Geometry check sheet. Reference: the model listing, model coordinates, mm. Face numbers are marked on the shaded views. A direction names the side the tool comes from. Coordinates: 2 decimals unless noted, no trailing zeros. Order: outer loops, then holes, each group sorted by start corner. A loop starts at its lowest first (then second) coordinate and runs counter-clockwise, first axis right, second up. Notation, with made-up numbers: M 65.25,-16.75 L 101.25,-16.75 A32 ccw 101.25,12.25 Z; hole C 39.25,54 d10. An arc over 180 degrees is marked long. One line per item, written item: value. Start each with the question number.
1) Thickness scan on L1, parallel to Z at x = 0, y = 2.8 (3 decimals); L2, parallel to Y at x = -5, z = 9; L3, parallel to Y at x = 12, z = 13. Record the ranges inside material, lowest first. Write a range as from..to.
2) Sectioned sample at D-D, the plane x = 10.5. Enter the section's corners in (y, z), then the cut area to 3 significant figures.
3) Sectioned sample at C-C, the plane y = 12.75. Enter the section's corners in (x, z) (3 decimals), then the cut area to 3 significant figures.
4) Access from +Z, -Z, +X, -X, +Y, -Y to the whole of each face (thin tool, end or side, straight path). Record for the marked faces 1, 2 and 3.
5) Sectioned sample at B-B, the plane y = 4.5. Enter the section's corners in (x, z) (3 decimals), then the cut area to 3 significant figures.
6) Sectioned sample at A-A, the plane z = 5.5. Enter the section's corners in (x, y) (3 decimals), then the cut area to 3 significant figures.
7) Go/stop test with flat-tipped pins: P1, Ø6, axis at y = 7.5, z = 6, coming from the -X side; P2, Ø1.5, axis at y = 2, z = 7, coming from the +X side; P3, Ø5, axis at x = -1.5, z = 4.5, coming from the +Y side; P4, Ø1.5, axis at x = 20, y = 4, coming from the -Z side. Record where each tip stops, or that it passes through.
8) Draft check along X on the marked faces 4, 5 and 6. Enter one of: pulls with the +X half, pulls with the -X half, needs draft (parallel to the pull), parting line crosses it, or undercut.
```python
from build123d import *

# Parameters (mm, degrees)
F1_DEPTH = 16
F2_R     = 3.125
F3_DEPTH = 10
F4_DEPTH = 5
F5_R     = 1
F6_R     = 1


with BuildPart() as f1:
    # F0 (on Top) → F1 (new body)
    with BuildSketch(Plane.XY):
        Polygon((-17.5, 15), (-30, 15), (-13, 0), (0, 0), (13, 0), (30, 15), (17.5, 15), (13, 10), (0, 10), (-13, 10), align=None)
    extrude(amount=F1_DEPTH)

    # F2 (on face) → F3 (cut, through all)
    with BuildSketch(Plane(origin=(0, 10, 0), x_dir=(-1, 0, 0), z_dir=(0, 1, 0))):
        with Locations((0, 8)):
            Circle(F2_R)
    extrude(amount=-F3_DEPTH, mode=Mode.SUBTRACT)

    # F2 (on face) → F4 (cut)
    with BuildSketch(Plane(origin=(0, 10, 0), x_dir=(-1, 0, 0), z_dir=(0, 1, 0))):
        Polygon((-5.86727, 11.34993), (-5.823923, 4.65007), (0, 1.33768), (5.780575, 4.72515), (5.737227, 11.42501), (-0.086695, 14.7374), align=None)
        with Locations((0, 8)):
            Circle(F2_R, mode=Mode.SUBTRACT)
    extrude(amount=-F4_DEPTH, mode=Mode.SUBTRACT)

    # F5
    f5_edges = [f1.edges().sort_by_distance(p)[0] for p in [
        (30, 15, 8),
    ]]
    fillet(f5_edges, radius=F5_R)

    # F6
    f6_edges = [f1.edges().sort_by_distance(p)[0] for p in [
        (-30, 15, 8),
    ]]
    fillet(f6_edges, radius=F6_R)


solid = f1.part
```
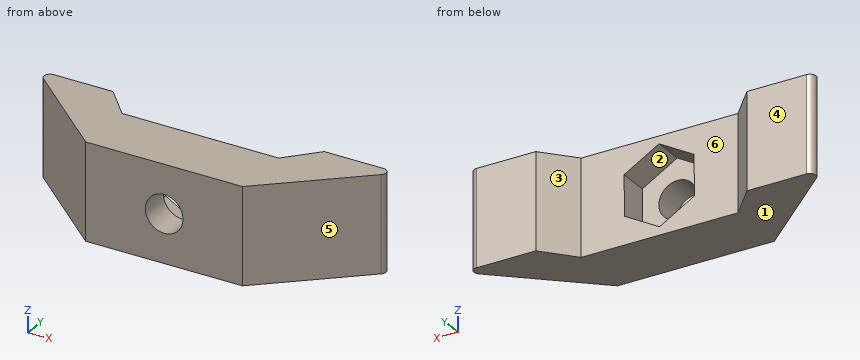
Final values:
1. L1: z = 0..4.875, 11.125..16
1. L2: y = 0..5
1. L3: y = 0..10
2. outline: M 0,0 L 10,0 L 10,16 L 0,16 Z
2. area: 160 mm^2
3. outline: M -27.45,0 L -15.475,0 L -15.475,16 L -27.45,16 Z; M 15.475,0 L 27.45,0 L 27.45,16 L 15.475,16 Z
3. area: 383 mm^2
4. face 1: -Z, +X, -X, +Y, -Y
4. face 2: +Y
4. face 3: +Z, -Z, +Y
5. outline: M -18.1,0 L 18.1,0 L 18.1,16 L -18.1,16 Z; hole C 0,8 d6.25
5. area: 549 mm^2
6. outline: M -28.017,13.25 L -13,0 L -1.875,0 L -1.875,5 L -5.776,5 L -5.776,10 L -13,10 L -17.5,15 L -27.355,15 A1 ccw Z; M 1.875,0 L 13,0 L 28.017,13.25 A1 ccw 27.355,15 L 17.5,15 L 13,10 L 5.829,10 L 5.829,5 L 1.875,5 Z
6. area: 413 mm^2
7. P1: stops at x = -24.9
7. P2: stops at x = 16.12
7. P3: stops at y = 10
7. P4: passes through
8. face 4: needs draft
8. face 5: pulls with the +X half
8. face 6: undercut
